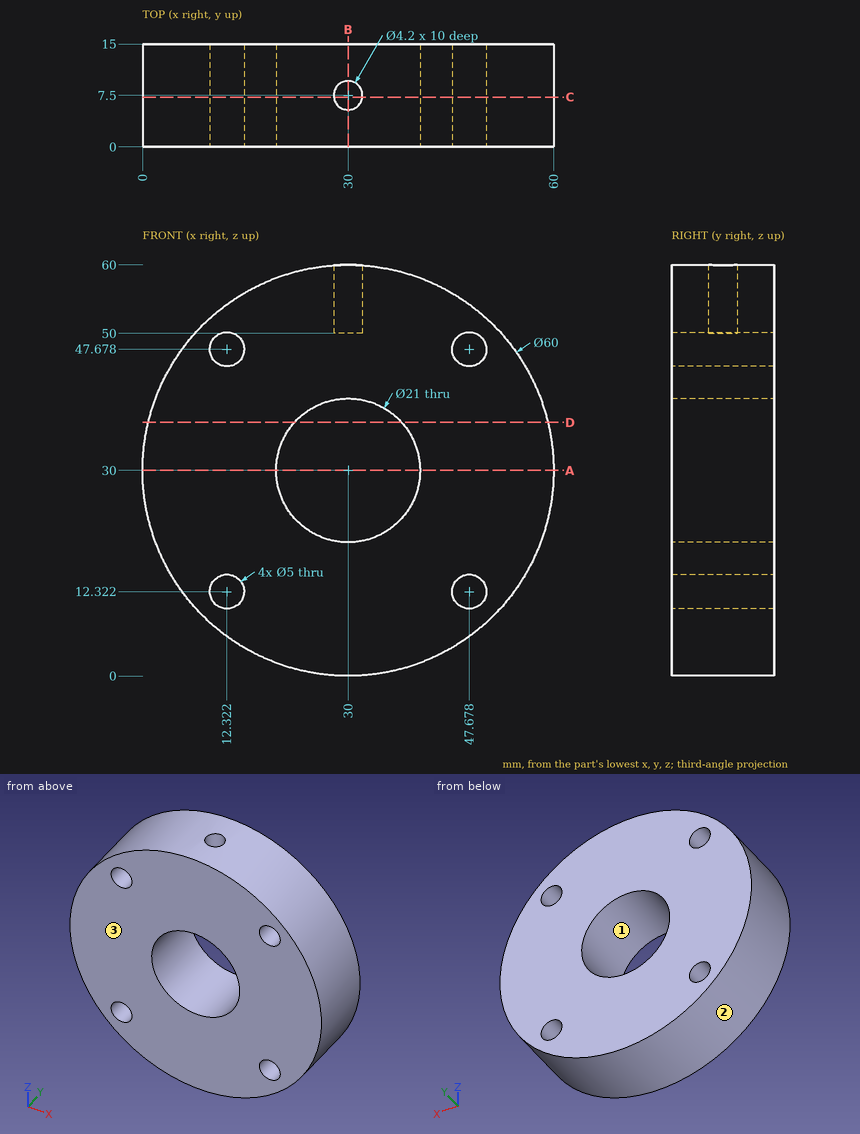
Here's the drawing with two shaded views (mm, measured from the low corner). I have some questions. Give positions to 0.01 mm unless a question says otherwise; leave off trailing zeros. Loops run counter-clockwise (first coordinate to the right, second up) from the corner with the lowest first, then second, coordinate; pieces in that order, holes last. Notation, with made-up numbers: (60.25, -22.5) -> (92.25, -22.5) arc R20 cw to (92.25, 1.5) -> close; hole circle Ø3 at (15, -8.75). An arc over 180 degrees is marked (long way). Answer as a JSON object with one key per item and string values. Group by question number.
Item 1: Imagine slicing it at D-D on z = 37. Write out the boundary of the cut face in (x, y).
Item 2: Imagine slicing it at C-C on y = 7.25. Write out the boundary of the cut face in (x, z) (1 decimal).
Item 3: Will these pins go through, and if not, where does the flat tip stop? pin 1 (2 mm diameter, centred on y = 6, z = 25, fed in from -X); pin 2 (8 mm diameter, centred on y = 11.5, z = 28, fed in from -X); pin 3 (4 mm diameter, centred on y = 2, z = 24.5, fed in from -X) (1 decimal).
Item 4: Imagine slicing it at A-A on z = 30. Write out the boundary of the cut face in (x, y), then the cut area to 3 significant figures.
Item 5: Thinking about a two-plate mould opening in X: for the marked faces 1, 2 and 3, which applies, pulls with the +X half, pulls with the -X half, needs draft (parallel to the pull), parting line crosses it, or undercut?
Item 6: I need wall thicknesses on L1, parallel to Z at x = 48, y = 8.25; L2, parallel to Z at x = 23, y = 11 (1 decimal). Which ranges of each line are inside material? Lowest first, please.
Item 7: Imagine slicing it at B-B on x = 30. Write out the boundary of the cut face in (y, z), then the cut area to 3 significant figures.
Answer list:
{
 "1": {"outline": "(0.83, 0) -> (22.17, 0) -> (22.17, 15) -> (0.83, 15) -> close; (37.83, 0) -> (59.17, 0) -> (59.17, 15) -> (37.83, 15) -> close"},
 "2": {"outline": "(27.9, 50) -> (27.9, 59.9) arc R30 ccw (long way) to (32.1, 59.9) -> (32.1, 50) -> close; hole circle Ø5 at (12.3, 12.3); hole circle Ø5 at (12.3, 47.7); hole circle Ø21 at (30, 30); hole circle Ø5 at (47.7, 12.3); hole circle Ø5 at (47.7, 47.7)"},
 "3": {"pin 1": "stops at x = 0.27", "pin 2": "stops at x = 0", "pin 3": "stops at x = 0.2"},
 "4": {"outline": "(0, 0) -> (19.5, 0) -> (19.5, 15) -> (0, 15) -> close; (40.5, 0) -> (60, 0) -> (60, 15) -> (40.5, 15) -> close", "area": "585 mm2"},
 "5": {"face 1": "undercut", "face 2": "parting line crosses it", "face 3": "needs draft"},
 "6": {"L1": "z = 6 to 9.84, 14.8 to 45.2, 50.16 to 54", "L2": "z = 0.8 to 22.2, 37.8 to 59.2"},
 "7": {"outline": "(0, 0) -> (15, 0) -> (15, 19.5) -> (0, 19.5) -> close; (0, 40.5) -> (15, 40.5) -> (15, 60) -> (9.6, 60) -> (9.6, 50) -> (5.4, 50) -> (5.4, 60) -> (0, 60) -> close", "area": "543 mm2"}
}
